Verification items for the finished model (mm, model axes). A direction names the side the tool comes from. Round coordinates to 2 decimals unless told otherwise and drop trailing zeros. Loops run counter-clockwise (first coordinate to the right, second up) from the corner with the lowest first, then second, coordinate; pieces in that order, holes last. Notation, with made-up numbers: M -19,36.5 L -2,36.5 A21 ccw -2,49.5 Z; hole C 73,-31.75 d9. An arc over 180 degrees is marked long. Write item = value, one per line. Start each with the question number.
from build123d import *

# Parameters (mm, degrees)
SKETCH_1_W                         = 46
SKETCH_1_H                         = 12
SKETCH_1_R                         = 2.25
SM_BASE_FLANGE_1_DEPTH             = 1.2
SM_EDGE_FLANGE_1_STRIP_W           = 6.2732
SM_EDGE_FLANGE_1_STRIP_H           = 1.2
SM_EDGE_FLANGE_1_STRIP_CUT_DEPTH   = 12
SM_EDGE_FLANGE_1_STRIP_2_W         = 6.2732
SM_EDGE_FLANGE_1_STRIP_2_H         = 1.2
SM_EDGE_FLANGE_1_STRIP_CUT_2_DEPTH = 12
SM_EDGE_FLANGE_1_DEPTH             = 12
SM_EDGE_FLANGE_1_BEND_DEPTH        = 12
SKETCH_12_R                        = 2.25
SKETCH_12_R_2                      = 1
CUT_EXTRUDE_1_DEPTH                = 52.121815304


# Sheet-metal steps are written as plain solids
with BuildPart() as part:
    # Sketch 1 → Базовая кромка1 (new body)
    with BuildSketch(Plane.XY):
        with Locations((23, 6)):
            Rectangle(SKETCH_1_W, SKETCH_1_H)
        with Locations((8, 6)):
            Circle(SKETCH_1_R, mode=Mode.SUBTRACT)
        with Locations((38, 6)):
            Circle(SKETCH_1_R, mode=Mode.SUBTRACT)
    extrude(amount=-SM_BASE_FLANGE_1_DEPTH)

    # Ребро-кромка1 strip (across the edge) → Ребро-кромка1 strip cut (cut)
    with BuildSketch(Plane.XZ.offset(-12)):
        with Locations((-1.2, -0.6)):
            Rectangle(SM_EDGE_FLANGE_1_STRIP_W, SM_EDGE_FLANGE_1_STRIP_H)
    extrude(amount=SM_EDGE_FLANGE_1_STRIP_CUT_DEPTH, mode=Mode.SUBTRACT)

    # Ребро-кромка1 strip 2 (across the edge) → Ребро-кромка1 strip cut 2 (cut)
    with BuildSketch(Plane(origin=(46, 0, 0), x_dir=(-1, 0, 0), z_dir=(0, 1, 0))):
        with Locations((-1.2, -0.6)):
            Rectangle(SM_EDGE_FLANGE_1_STRIP_2_W, SM_EDGE_FLANGE_1_STRIP_2_H)
    extrude(amount=SM_EDGE_FLANGE_1_STRIP_CUT_2_DEPTH, mode=Mode.SUBTRACT)

    # Ребро-кромка1 section (across the edge) → Ребро-кромка1 (add)
    with BuildSketch(Plane.XZ.offset(-12)):
        with BuildLine():
            Line((0, 0.7366), (0, 18.8))
            Line((0, 18.8), (1.2, 18.8))
            Line((1.2, 18.8), (1.2, 0.7366))
            ThreePointArc((1.2, 0.7366), (1.415745145, 0.215745145), (1.9366, 0))
            Line((1.9366, 0), (1.9366, -1.2))
            ThreePointArc((1.9366, -1.2), (0.567217008, -0.632782992), (0, 0.7366))
        make_face()
    extrude(amount=SM_EDGE_FLANGE_1_DEPTH)

    # Ребро-кромка1 section 2 (across the edge) → Ребро-кромка1 bend (add)
    with BuildSketch(Plane(origin=(46, 0, 0), x_dir=(-1, 0, 0), z_dir=(0, 1, 0))):
        with BuildLine():
            Line((0, 0.7366), (0, 18.8))
            Line((0, 18.8), (1.2, 18.8))
            Line((1.2, 18.8), (1.2, 0.7366))
            ThreePointArc((1.2, 0.7366), (1.415745145, 0.215745145), (1.9366, 0))
            Line((1.9366, 0), (1.9366, -1.2))
            ThreePointArc((1.9366, -1.2), (0.567217008, -0.632782992), (0, 0.7366))
        make_face()
    extrude(amount=SM_EDGE_FLANGE_1_BEND_DEPTH)

    # Эскиз12 → Вырез-Вытянуть1 (cut, through all)
    with BuildSketch(Plane(origin=(46, 0, 0), x_dir=(0, 0, -1), z_dir=(1, 0, 0))):
        with Locations((-14.3, 6)):
            Circle(SKETCH_12_R)
        with Locations((-7.3, 6)):
            Circle(SKETCH_12_R_2)
        with Locations((-2.3, 6)):
            Circle(SKETCH_12_R_2)
    extrude(amount=-CUT_EXTRUDE_1_DEPTH, mode=Mode.SUBTRACT)


solid = part.part
1. Section check D-D, the plane z = 2.3. Enter the section's corners in (x, y).
2. Mould release check, pull along Z, two halves, no side actions. Record for faces 1 (the cylindrical face through (45.408, 6.676, 3.037)), 2 (the cylindrical face through (5.752, 6.099, -0.592)), 3 (the cylindrical face through (0.582, 6.084, -0.648)): pulls with the +Z half, pulls with the -Z half, needs draft (parallel to the pull), parting line crosses it, or undercut.
3. Section check B-B, the plane x = 8. Enter the section's corners in (y, z).
4. Section check C-C, the plane y = 10.5. Enter the section's corners in (x, z), and give its area (3 significant figures).
5. Tool access check on faces 4 (the cylindrical face through (0.608, 6.099, 16.548)), 5 (the flat face through (23, 6, 0)). Record the directions out of +Z, -Z, +X, -X, +Y, -Y that give a thin tool (end or side, any length) a straight path to the whole face; none if there is none.
6. Thickness scan on line 1 (X direction, y = 2.5, z = 3.25); line 2 (Y direction, x = 0.65, z = 14.3); line 3 (Y direction, x = 0.45, z = 7.3). Record the ranges inside material, lowest first.
7. Gauge pin test, flat ends, axial feed: P1, Ø4, axis at x = 38, y = 6, coming from the -Z side; P2, Ø1, axis at x = 26, y = 2.5, coming from the +Z side. Record the tip position at first contact, or that the pin passes through.
8. Section check A-A, the plane z = 14.3. Enter the section's corners in (x, y).
Computed values:
q1.outline = M 0,0 L 1.2,0 L 1.2,5 L 0,5 Z; M 0,7 L 1.2,7 L 1.2,12 L 0,12 Z; M 44.8,0 L 46,0 L 46,5 L 44.8,5 Z; M 44.8,7 L 46,7 L 46,12 L 44.8,12 Z
q2.face_1 = undercut
q2.face_2 = needs draft
q2.face_3 = pulls with the -Z half
q3.outline = M 0,-1.2 L 3.75,-1.2 L 3.75,0 L 0,0 Z; M 8.25,-1.2 L 12,-1.2 L 12,0 L 8.25,0 Z
q4.outline = M 0,0.74 A1.94 ccw 1.94,-1.2 L 44.06,-1.2 A1.94 ccw 46,0.74 L 46,18.8 L 44.8,18.8 L 44.8,0.74 A0.74 cw 44.06,0 L 1.94,0 A0.74 cw 1.2,0.74 L 1.2,18.8 L 0,18.8 Z
q4.area = 98.9 mm2
q5.face_4 = +X, -X
q5.face_5 = +Z, +Y, -Y
q6.line_1 = 0 to 1.2, 44.8 to 46
q6.line_2 = 0 to 3.75, 8.25 to 12
q6.line_3 = 0 to 5, 7 to 12
q7.P1 = through
q7.P2 = 0
q8.outline = M 0,0 L 1.2,0 L 1.2,3.75 L 0,3.75 Z; M 0,8.25 L 1.2,8.25 L 1.2,12 L 0,12 Z; M 44.8,0 L 46,0 L 46,3.75 L 44.8,3.75 Z; M 44.8,8.25 L 46,8.25 L 46,12 L 44.8,12 Z
